from build123d import *

# Parameters (mm, degrees)
SKETCH1_W           = 22.5
SKETCH1_H           = 8
SKETCH1_R           = 1.47
BOSS_EXTRUDE1_DEPTH = 1.59
CUT_EXTRUDE1_DEPTH  = 13.3561685


with BuildPart() as part:
    # Sketch1 → Boss-Extrude1 (new, symmetric)
    with BuildSketch(Plane.XY):
        Rectangle(SKETCH1_W, SKETCH1_H)
        with Locations(Location((-9.5, 0, 0), (0, 0, 180))):
            Circle(SKETCH1_R, mode=Mode.SUBTRACT)
    extrude(amount=BOSS_EXTRUDE1_DEPTH, both=True)

    # Sketch2 → Cut-Extrude1 (cut, through all)
    with BuildSketch(Plane(origin=(0, 0, -1.59), x_dir=(-1, 0, 0), z_dir=(0, 0, -1))):
        Polygon((-3.39, -1.475), (-1.32, -1.475), (-1.32, 1.475), (-3.39, 1.475), (-3.39, 3.25), (-5.99, 3.25), (-5.99, 1.475), (-8.07, 1.475), (-8.07, 2.5), (-11.25, 2.5), (-11.25, -2.5), (-8.07, -2.5), (-8.07, -1.475), (-5.99, -1.475), (-5.99, -3.25), (-3.39, -3.25), align=None)
    extrude(amount=-CUT_EXTRUDE1_DEPTH, mode=Mode.SUBTRACT)


solid = part.part
Check sheet for the modelled part. Datum: model origin and axes. Units: mm. A direction names the side the tool comes from. Give positions to 0.01 mm unless a question says otherwise; leave off trailing zeros. Write each loop counter-clockwise with the first axis right and the second up, starting at its lowest first coordinate (ties: lowest second). Pieces come first, ordered by that corner, then holes. Notation, with made-up numbers: (44.25, 54) -> (88.25, 54) arc R22 ccw to (88.25, 64) -> close; hole circle Ø1 at (73, 71). An arc over 180 degrees is marked (long way). Write item = value, one per line.
Item 1: Sectioned sample at A-A on x = 2.5. Record the boundary of the cut face in (y, z) (3 decimals), and give its area (3 significant figures).
Output:
outline = (-4, -1.59) -> (-1.475, -1.59) -> (-1.475, 1.59) -> (-4, 1.59) -> close; (1.475, -1.59) -> (4, -1.59) -> (4, 1.59) -> (1.475, 1.59) -> close
area = 16.1 mm^2
Item 2: Tool access check on faces 4 (the flat face through (3.39, 2, 0)), 5 (the flat face through (10, 2.5, 0)), 6 (the flat face through (11.25, 3, 0)). Record the directions out of +Z, -Z, +X, -X, +Y, -Y that give a thin tool (end or side, any length) a straight path to the whole face; none if there is none.
Output:
face_4 = +Z, -Z
face_5 = +Z, -Z, +X
face_6 = +Z, -Z, +X, +Y, -Y
Item 3: Gauge pin test, flat end, axial feed: pin 1 (0.9 mm diameter, centred on y = -0.5, z = -0.5, fed in from +X). Record the tip position at first contact, or that the pin passes through.
Output:
pin_1 = 1.32
Item 4: Release check for a two-part mould opening along Y. For faces 1 (the flat face through (-3, 0, -1.59)), 2 (the flat face through (0, 4, 0)), 3 (the flat face through (10, -2.5, 0)) record: +Y half, -Y half, draft (parallel to the pull), parting line (faces both ways), or undercut.
Output:
face_1 = draft
face_2 = +Y half
face_3 = undercut
Item 5: Sectioned sample at C-C on z = 0.6. Record the boundary of the cut face in (x, y) (3 decimals), and give its area (3 significant figures).
Output:
outline = (-11.25, -4) -> (11.25, -4) -> (11.25, -2.5) -> (8.07, -2.5) -> (8.07, -1.475) -> (5.99, -1.475) -> (5.99, -3.25) -> (3.39, -3.25) -> (3.39, -1.475) -> (1.32, -1.475) -> (1.32, 1.475) -> (3.39, 1.475) -> (3.39, 3.25) -> (5.99, 3.25) -> (5.99, 1.475) -> (8.07, 1.475) -> (8.07, 2.5) -> (11.25, 2.5) -> (11.25, 4) -> (-11.25, 4) -> close; hole circle Ø2.94 at (-9.5, 0)
area = 128 mm^2
Item 6: Sectioned sample at B-B on y = 0. Record the boundary of the cut face in (x, z).
Output:
outline = (-11.25, -1.59) -> (-10.97, -1.59) -> (-10.97, 1.59) -> (-11.25, 1.59) -> close; (-8.03, -1.59) -> (1.32, -1.59) -> (1.32, 1.59) -> (-8.03, 1.59) -> close
Item 7: Scan lines: probe 1 along Y at (x, z) = (-9.5, -0.6); probe 2 along Y at (x, z) = (4.25, 0.45); probe 3 along X at (y, z) = (2.25, -1.1). Record each from-to range of solid material in increasing order. Write a range as from..to.
Output:
probe_1 = -4..-1.47, 1.47..4
probe_2 = -4..-3.25, 3.25..4
probe_3 = -11.25..3.39, 5.99..8.07
